For this review, take the finished solid that the model builds, in its own axes (mm). A direction names the side the tool comes from. Coordinates: 2 decimals unless noted, no trailing zeros. Loops run counter-clockwise (first coordinate to the right, second up) from the corner with the lowest first, then second, coordinate; pieces in that order, holes last. Notation, with made-up numbers: M 34,63.5 L 64,63.5 A27 cw 64,81.5 Z; hole C 69.5,-2.5 d8. An arc over 180 degrees is marked long. Write item = value, one per line.
from build123d import *

# Parameters (mm, degrees)
SKETCH1_W           = 137.4
SKETCH1_H           = 88
BOSS_EXTRUDE1_DEPTH = 3
SKETCH2_R           = 1.75
CUT_EXTRUDE1_DEPTH  = 4
SKETCH3_W           = 9
SKETCH3_H           = 3.8
SKETCH3_W_2         = 3.8
SKETCH3_H_2         = 10
BOSS_EXTRUDE2_DEPTH = 3
SKETCH4_R           = 3.75
CUT_EXTRUDE2_DEPTH  = 4


with BuildPart() as part:
    # Sketch1 → Boss-Extrude1 (new body)
    with BuildSketch(Plane(origin=(0, 0, 0), x_dir=(1, 0, 0), z_dir=(0, 1, 0))):
        with Locations((68.7, -44)):
            Rectangle(SKETCH1_W, SKETCH1_H)
    extrude(amount=BOSS_EXTRUDE1_DEPTH)

    # Sketch2 → Cut-Extrude1 (cut, through all)
    with BuildSketch(Plane.XZ):
        with Locations((3, 85)):
            Circle(SKETCH2_R)
        with Locations((134.4, 85)):
            Circle(SKETCH2_R)
        with Locations((134.4, 3)):
            Circle(SKETCH2_R)
        with Locations((3, 3)):
            Circle(SKETCH2_R)
    extrude(amount=-CUT_EXTRUDE1_DEPTH, mode=Mode.SUBTRACT)

    # Sketch3 → Boss-Extrude2 (add, through all)
    with BuildSketch(Plane.XZ):
        Polygon((0, 91.8), (-3.8, 91.8), (-3.8, 78), (0, 78), (0, 88), align=None)
        with Locations((4.5, 89.9)):
            Rectangle(SKETCH3_W, SKETCH3_H)
        with Locations((-1.9, 5)):
            Rectangle(SKETCH3_W_2, SKETCH3_H_2)
        Polygon((9, 0), (0, 0), (-3.8, 0), (-3.8, -3.8), (9, -3.8), align=None)
        Polygon((137.4, 0), (128.4, 0), (128.4, -3.8), (141.2, -3.8), (141.2, 0), align=None)
        with Locations((139.3, 5)):
            Rectangle(SKETCH3_W_2, SKETCH3_H_2)
        with Locations((132.9, 89.9)):
            Rectangle(SKETCH3_W, SKETCH3_H)
        Polygon((137.4, 91.8), (137.4, 88), (137.4, 78), (141.2, 78), (141.2, 91.8), align=None)
    extrude(amount=-BOSS_EXTRUDE2_DEPTH)

    # Sketch4 → Cut-Extrude2 (cut, through all)
    with BuildSketch(Plane.XZ):
        with Locations((24.5, 47.5)):
            Circle(SKETCH4_R)
        with Locations((24.5, 27.75)):
            Circle(SKETCH4_R)
    extrude(amount=-CUT_EXTRUDE2_DEPTH, mode=Mode.SUBTRACT)


solid = part.part
Q1. Draft analysis for pull direction X (two halves, no side actions). For faces 6 (the face through (128.4, 1, 90)), 7 (the face through (3, 1, -3.8)), 8 (the face through (141.2, 1, 3)), state which applies: +X half, -X half, draft (parallel to the pull), parting line (faces both ways), or undercut.
Solved:
face_6 = undercut
face_7 = draft
face_8 = +X half
Q2. Add section D-D (z = 47.5). Write out the cut boundary in (x, y), and give its area (3 significant figures).
Solved:
outline = M 0,0 L 20.75,0 L 20.75,3 L 0,3 Z; M 28.25,0 L 137.4,0 L 137.4,3 L 28.25,3 Z
area = 390 mm²
Q3. For line 1 along Z through (x, y) = (3, 2.35); line 2 along X through (y, z) = (2.25, 85); line 3 along Z through (x, y) = (24.5, 1.4), list the stretches that pass through material, from the lowest coordinate up.
Solved:
line_1 = -3.8 to 1.25, 4.75 to 83.25, 86.75 to 91.8
line_2 = -3.8 to 1.25, 4.75 to 132.65, 136.15 to 141.2
line_3 = 0 to 24, 31.5 to 43.75, 51.25 to 88
Q4. For pin 1 Ø0.9 at (x, y) = (92, 1.5) entering from -Z; pin 2 Ø0.9 at (x, y) = (45.5, 2) entering from +Z, all flat-tipped, find the tip position at first contact; note any pin that passes through.
Solved:
pin_1 = 0
pin_2 = 88
Q5. Add section C-C (x = 24.5). Write out the cut boundary in (y, z), and give its area (3 significant figures).
Solved:
outline = M 0,0 L 3,0 L 3,24 L 0,24 Z; M 0,31.5 L 3,31.5 L 3,43.75 L 0,43.75 Z; M 0,51.25 L 3,51.25 L 3,88 L 0,88 Z
area = 219 mm²
Q6. Machinability: for faces 1 (the face through (26.23, 1.479, 44.173)), 2 (the face through (-2, 1, 10)), 3 (the face through (9, 1, 90)), 4 (the face through (68, 1, 0)), 5 (the face through (139, 1, 78)), which of the approach directions +Z, -Z, +X, -X, +Y, -Y give a long, thin tool a straight path to every point of the face, cutting with its end or side? Answer none if there is none.
Solved:
face_1 = +Y, -Y
face_2 = -X, +Y, -Y
face_3 = +Z, +Y, -Y
face_4 = -Z, +Y, -Y
face_5 = +X, +Y, -Y
Q7. Add section A-A (z = 3). Write out the cut boundary in (x, y), and give its area (3 significant figures).
Solved:
outline = M -3.8,0 L 1.25,0 L 1.25,3 L -3.8,3 Z; M 4.75,0 L 132.65,0 L 132.65,3 L 4.75,3 Z; M 136.15,0 L 141.2,0 L 141.2,3 L 136.15,3 Z
area = 414 mm²
Q8. Add section B-B (y = 2.55). Write out the cut boundary in (x, z).
Solved:
outline = M -3.8,-3.8 L 9,-3.8 L 9,0 L 128.4,0 L 128.4,-3.8 L 141.2,-3.8 L 141.2,10 L 137.4,10 L 137.4,78 L 141.2,78 L 141.2,91.8 L 128.4,91.8 L 128.4,88 L 9,88 L 9,91.8 L -3.8,91.8 L -3.8,78 L 0,78 L 0,10 L -3.8,10 Z; hole C 3,3 d3.5; hole C 3,85 d3.5; hole C 24.5,27.75 d7.5; hole C 24.5,47.5 d7.5; hole C 134.4,3 d3.5; hole C 134.4,85 d3.5
